```python
from build123d import *

# Parameters (mm, degrees)
SKETCH1_W           = 50
SKETCH1_H           = 25
BOSS_EXTRUDE1_DEPTH = 170
SKETCH2_R           = 7.5
CUT_EXTRUDE1_DEPTH  = 179.955301682
SKETCH3_R           = 7.5
CUT_EXTRUDE2_DEPTH  = 170


with BuildPart() as part:
    # Sketch1 → Boss-Extrude1 (new body)
    with BuildSketch(Plane.XY):
        with Locations((25, -12.5)):
            Rectangle(SKETCH1_W, SKETCH1_H)
    extrude(amount=BOSS_EXTRUDE1_DEPTH)

    # Sketch2 → Cut-Extrude1 (cut, through all)
    with BuildSketch(Plane(origin=(0, 0, 0), x_dir=(1, 0, 0), z_dir=(0, 1, 0))):
        with Locations(Location((25, -20, 0), (0, 0, 180))):
            Circle(SKETCH2_R)
    extrude(amount=-CUT_EXTRUDE1_DEPTH, mode=Mode.SUBTRACT)

    # Sketch3 → Cut-Extrude2 (cut)
    with BuildSketch(Plane(origin=(0, 0, 0), x_dir=(1, 0, 0), z_dir=(0, 1, 0))):
        with Locations(Location((25, -150, 0), (0, 0, 270))):
            Circle(SKETCH3_R)
    extrude(amount=-CUT_EXTRUDE2_DEPTH, mode=Mode.SUBTRACT)


solid = part.part
```
The listing builds one solid part. Answer for the finished solid, in the listing's coordinates (mm). Coordinates: 2 decimals unless noted, no trailing zeros. Write each loop counter-clockwise with the first axis right and the second up, starting at its lowest first coordinate (ties: lowest second). Pieces come first, ordered by that corner, then holes. Notation, with made-up numbers: (68.25, -39.75) - (76.25, -39.75) arc R25 cw to (76.25, -20.75) - close; hole circle Ø10 at (14.25, -35.75). An arc over 180 degrees is marked (long way). One line per item, written item: value.
1) For a pull along X with two mould halves and no side action, classify faces 1 (the cylindrical face through (27.253, -12.325, 157.154)), 2 (the flat face through (25, -12, 170)), 3 (the flat face through (50, -13, 84)) as pulls with the +X half, pulls with the -X half, needs draft (parallel to the pull), parting line crosses it, or undercut.
Geometry check:
face 1: undercut
face 2: needs draft
face 3: pulls with the +X half
2) This flat-tipped pin is pushed along its axis until it touches: pin 1 Ø3 at (y, z) = (-4, 80) entering from -X. Where does it stop, or does it pass through?
Geometry check:
pin 1: stops at x = 0
3) Consider line 1 along X through (y, z) = (-6.75, 150); line 2 along Z through (x, y) = (26, -16.5); line 3 along Z through (x, y) = (23.5, -5.25). Determine where each line is inside the solid, lowest interval first. Write a range as from..to.
Geometry check:
line 1: x = 0..17.5, 32.5..50
line 2: z = 0..12.57, 27.43..142.57, 157.43..170
line 3: z = 0..12.65, 27.35..142.65, 157.35..170
4) Find section B-B (z = 150). Give the vertices of the cut face in (x, y), and give its area (3 significant figures).
Geometry check:
outline: (0, -25) - (17.5, -25) - (17.5, 0) - (0, 0) - close; (32.5, -25) - (50, -25) - (50, 0) - (32.5, 0) - close
area: 875 mm2
5) Find section A-A (x = 25). Give the vertices of the cut face in (y, z), and give its area (3 significant figures).
Geometry check:
outline: (-25, 0) - (0, 0) - (0, 12.5) - (-25, 12.5) - close; (-25, 27.5) - (0, 27.5) - (0, 142.5) - (-25, 142.5) - close; (-25, 157.5) - (0, 157.5) - (0, 170) - (-25, 170) - close
area: 3,500 mm2
6) Find section C-C (y = -11.5). Give the vertices of the cut face in (x, z).
Geometry check:
outline: (0, 0) - (50, 0) - (50, 170) - (0, 170) - close; hole circle Ø15 at (25, 20); hole circle Ø15 at (25, 150)
